Work out the finished part from the listing and answer in its coordinate system (mm). A direction names the side the tool comes from. Round coordinates to 2 decimals unless told otherwise and drop trailing zeros. Loops run counter-clockwise (first coordinate to the right, second up) from the corner with the lowest first, then second, coordinate; pieces in that order, holes last.
```python
from build123d import *

# Parameters (mm, degrees)
BOSS_EXTRUDE1_DEPTH     = 3.175
CUT_EXTRUDE1_DEPTH      = 136.62296533
CUT_EXTRUDE1_DEPTH_BACK = 136.62296533
SKETCH2_R               = 1.6


with BuildPart() as part:
    # Sketch1 → Boss-Extrude1 (new body)
    with BuildSketch(Plane(origin=(0, 0, 0), x_dir=(1, 0, 0), z_dir=(0, 1, 0))):
        Polygon((-12.5875, 0), (12.5875, 0), (12.5875, -55), (9.415, -55), (9.415, -88), (12.59, -88), (12.59, -108), (9.415, -108), (9.415, -135), (-9.415, -135), (-9.415, -108), (-12.59, -108), (-12.59, -88), (-9.415, -88), (-9.415, -55), (-12.5875, -55), align=None)
    extrude(amount=BOSS_EXTRUDE1_DEPTH)

    # Sketch2 → Cut-Extrude1 (cut, two sides: drawn at the far end of the back side and taken through both)
    with BuildSketch(Plane(origin=(0, 3.175, 0), x_dir=(1, 0, 0), z_dir=(0, 1, 0)).offset(-CUT_EXTRUDE1_DEPTH_BACK)):
        with Locations(Location((0, -24, 0), (0, 0, 270))):
            Circle(SKETCH2_R)
        with Locations(Location((0, -12, 0), (0, 0, 270))):
            Circle(SKETCH2_R)
    extrude(amount=CUT_EXTRUDE1_DEPTH + CUT_EXTRUDE1_DEPTH_BACK, mode=Mode.SUBTRACT)


solid = part.part
```
1. Find section A-A (x = 0). Write down the section's boundary in (y, z) (3 decimals).
Answer key:
outline: (0, 0) - (3.175, 0) - (3.175, 10.4) - (0, 10.4) - close; (0, 13.6) - (3.175, 13.6) - (3.175, 22.4) - (0, 22.4) - close; (0, 25.6) - (3.175, 25.6) - (3.175, 135) - (0, 135) - close
2. Consider probe 1 along Z at (x, y) = (0, 1.4); probe 2 along Z at (x, y) = (-11.25, 0.9); probe 3 along X at (y, z) = (2, 24). Determine where each line is inside the solid, lowest interval first.
Answer key:
probe 1: z = 0 to 10.4, 13.6 to 22.4, 25.6 to 135
probe 2: z = 0 to 55, 88 to 108
probe 3: x = -12.59 to -1.6, 1.6 to 12.59
3. Which of the six approach directions +Z, -Z, +X, -X, +Y, -Y give full straight-line access (tool end or side, diameter ignored) to faces 1 (the face through (-11, 2, 108)), 2 (the face through (11, 2, 55)), 3 (the face through (11, 2, 108))?
Answer key:
face 1: +Z, -X, +Y, -Y
face 2: +X, +Y, -Y
face 3: +Z, +X, +Y, -Y
4. Find section C-C (z = 24). Write down the section's boundary in (x, y) (1 decimal).
Answer key:
outline: (-12.6, 0) - (-1.6, 0) - (-1.6, 3.2) - (-12.6, 3.2) - close; (1.6, 0) - (12.6, 0) - (12.6, 3.2) - (1.6, 3.2) - close
5. Find section D-D (z = 124). Write down the section's boundary in (x, y) (3 decimals), then the cut area to 3 significant figures.
Answer key:
outline: (-9.415, 0) - (9.415, 0) - (9.415, 3.175) - (-9.415, 3.175) - close
area: 59.8 mm2
6. Given pin 1 (1 mm diameter, centred on y = 2.5, z = 71.5, fed in from -X) (3 decimals); pin 2 (1.6 mm diameter, centred on y = 2, z = 64.5, fed in from +X) (3 decimals); pin 3 (1 mm diameter, centred on y = 2.5, z = 34, fed in from -X), each flat-ended and moving along its own axis, determine where each tip first touches the part or whether it passes through.
Answer key:
pin 1: stops at x = -9.415
pin 2: stops at x = 9.415
pin 3: stops at x = -12.59
7. Find section B-B (y = 2.3). Write down the section's boundary in (x, z) (1 decimal).
Answer key:
outline: (-12.6, 0) - (12.6, 0) - (12.6, 55) - (9.4, 55) - (9.4, 88) - (12.6, 88) - (12.6, 108) - (9.4, 108) - (9.4, 135) - (-9.4, 135) - (-9.4, 108) - (-12.6, 108) - (-12.6, 88) - (-9.4, 88) - (-9.4, 55) - (-12.6, 55) - close; hole circle Ø3.2 at (0, 12); hole circle Ø3.2 at (0, 24)
8. Determine the mould class of faces 4 (the face through (0, 2, 135)), 5 (the face through (9.415, 2, 121)), 6 (the face through (-11, 2, 88)) for opening direction Z: +Z half, -Z half, draft (parallel to the pull), parting line (faces both ways), or undercut.
Answer key:
face 4: +Z half
face 5: draft
face 6: undercut
